```python
from build123d import *

# Parameters (mm, degrees)
SKETCH1_R           = 11
SKETCH1_R_2         = 1.6
BOSS_EXTRUDE1_DEPTH = 5.5
SKETCH2_R           = 3.25
BOSS_EXTRUDE3_DEPTH = 9
CUT_EXTRUDE2_START  = -8
CUT_EXTRUDE2_DEPTH  = 8
SKETCH5_R           = 1.5
CUT_EXTRUDE3_DEPTH  = 22.266170318
CHAMFER1_SIZE       = 1.25
CHAMFER1_SIZE2      = 0.721687836


with BuildPart() as part:
    # Sketch1 → Boss-Extrude1 (new body)
    with BuildSketch(Plane(origin=(0, 0, 0), x_dir=(1, 0, 0), z_dir=(0, 1, 0))):
        with Locations(Location((0, 0, 0), (0, 0, 270))):
            Circle(SKETCH1_R)
        with Locations(Location((0, 7.9, 0), (0, 0, 270))):
            Circle(SKETCH1_R_2, mode=Mode.SUBTRACT)
        with Locations(Location((7.9, 0, 0), (0, 0, 270))):
            Circle(SKETCH1_R_2, mode=Mode.SUBTRACT)
        with Locations(Location((0, -7.9, 0), (0, 0, 270))):
            Circle(SKETCH1_R_2, mode=Mode.SUBTRACT)
        with Locations(Location((-7.9, 0, 0), (0, 0, 270))):
            Circle(SKETCH1_R_2, mode=Mode.SUBTRACT)
    extrude(amount=BOSS_EXTRUDE1_DEPTH)

    # Sketch2 → Boss-Extrude3 (add)
    with BuildSketch(Plane(origin=(0, 5.5, 0), x_dir=(1, 0, 0), z_dir=(0, 1, 0))):
        with Locations(Location((0, 0, 0), (0, 0, 270))):
            Circle(SKETCH2_R)
    extrude(amount=BOSS_EXTRUDE3_DEPTH)

    # Sketch4 → Cut-Extrude2 (cut)
    with BuildSketch(Plane(origin=(0, 14.5, 0), x_dir=(1, 0, 0), z_dir=(0, 1, 0)).offset(CUT_EXTRUDE2_START)):
        with BuildLine():
            Line((2.5, -2.076655966), (-2.5, -2.076655966))
            ThreePointArc((-2.5, -2.076655966), (0, -3.25), (2.5, -2.076655966))
        make_face()
    extrude(amount=CUT_EXTRUDE2_DEPTH, mode=Mode.SUBTRACT)

    # Sketch5 → Cut-Extrude3 (cut, through all)
    with BuildSketch(Plane(origin=(0, 14.5, 0), x_dir=(1, 0, 0), z_dir=(0, 1, 0))):
        with Locations(Location((0, 0, 0), (0, 0, 270))):
            Circle(SKETCH5_R)
    extrude(amount=-CUT_EXTRUDE3_DEPTH, mode=Mode.SUBTRACT)

    # Chamfer1
    chamfer1_edges = [part.edges().sort_by_distance(p)[0] for p in [
        (0, 0, -1.5),
    ]]
    chamfer1_side = [part.faces().sort_by_distance(p)[0] for p in [
        (0, 0, -10.688873016),
    ]]
    chamfer(chamfer1_edges, length=CHAMFER1_SIZE, length2=CHAMFER1_SIZE2, reference=chamfer1_side[0])


solid = part.part
```
Geometry check sheet. Reference: the model listing, model coordinates, mm. A direction names the side the tool comes from. Give positions to 0.01 mm unless a question says otherwise; leave off trailing zeros. Loops run counter-clockwise (first coordinate to the right, second up) from the corner with the lowest first, then second, coordinate; pieces in that order, holes last. Notation, with made-up numbers: M 14.5,66.5 L 55.5,66.5 A11 cw 55.5,86.5 Z; hole C 61.5,6 d5. An arc over 180 degrees is marked long. Write item = value, one per line.
(1) Sectioned sample at A-A, the plane x = 0. Record the cut outline in (y, z).
Answer below:
outline = M 0,-11 L 5.5,-11 L 5.5,-9.5 L 0,-9.5 Z; M 0,-6.3 L 5.5,-6.3 L 5.5,-3.25 L 14.5,-3.25 L 14.5,-1.5 L 0.72,-1.5 L 0,-2.75 Z; M 0,2.75 L 0.72,1.5 L 14.5,1.5 L 14.5,2.08 L 6.5,2.08 L 6.5,3.25 L 5.5,3.25 L 5.5,6.3 L 0,6.3 Z; M 0,9.5 L 5.5,9.5 L 5.5,11 L 0,11 Z
(2) Tool access check on faces 1 (the face through (0, 10, 2.077)), 2 (the face through (9.25, 2.71, 0.86)), 3 (the face through (-2, 5.5, -3)). Record the directions out of +Z, -Z, +X, -X, +Y, -Y that give a thin tool (end or side, any length) a straight path to the whole face; none if there is none.
Answer below:
face_1 = +Z, +X, -X, +Y
face_2 = +Y, -Y
face_3 = +Y
(3) Sectioned sample at D-D, the plane x = -7.9. Record the cut outline in (y, z).
Answer below:
outline = M 0,-7.65 L 5.5,-7.65 L 5.5,-1.6 L 0,-1.6 Z; M 0,1.6 L 5.5,1.6 L 5.5,7.65 L 0,7.65 Z
(4) Release check for a two-part mould opening along Z. For faces 4 (the face through (-0.61, 2.71, 9.38)), 5 (the face through (0, 6.5, 3)), 6 (the face through (0.143, 9.937, -3.247)) record: released by +Z, released by -Z, zero draft, split by the parting line, or undercut.
Answer below:
face_4 = undercut
face_5 = zero draft
face_6 = split by the parting line
(5) Gauge pin test, flat ends, axial feed: pin 1 Ø6 at (x, y) = (3, 11.5) entering from +Z; pin 2 Ø1 at (x, z) = (-5, -0.5) entering from -Y; pin 3 Ø3 at (x, y) = (-0.5, 7.5) entering from +Z; pin 4 Ø5 at (x, y) = (-3.5, 3) entering from -Z. Record the tip position at first contact, or that the pin passes through.
Answer below:
pin_1 = 2.08
pin_2 = 0
pin_3 = 3.25
pin_4 = -10.95
(6) Sectioned sample at B-B, the plane z = 0. Record the cut outline in (x, y), plus the area to 3 significant figures.
Answer below:
outline = M -11,0 L -9.5,0 L -9.5,5.5 L -11,5.5 Z; M -6.3,0 L -2.75,0 L -1.5,0.72 L -1.5,14.5 L -3.25,14.5 L -3.25,5.5 L -6.3,5.5 Z; M 1.5,0.72 L 2.75,0 L 6.3,0 L 6.3,5.5 L 3.25,5.5 L 3.25,14.5 L 1.5,14.5 Z; M 9.5,0 L 11,0 L 11,5.5 L 9.5,5.5 Z
area = 99.9 mm2
(7) Sectioned sample at C-C, the plane z = -7.9. Record the cut outline in (x, y).
Answer below:
outline = M -7.65,0 L -1.6,0 L -1.6,5.5 L -7.65,5.5 Z; M 1.6,0 L 7.65,0 L 7.65,5.5 L 1.6,5.5 Z
(8) Material ranges on line 1 (X direction, y = 3.45, z = 0); line 2 (Y direction, x = 3.5, z = -6); line 3 (Z direction, x = 0.75, y = 1.5), recorded low to high. Write a range as [from, to].
Answer below:
line_1 = [-11, -9.5], [-6.3, -1.5], [1.5, 6.3], [9.5, 11]
line_2 = [0, 5.5]
line_3 = [-10.97, -9.31], [-6.49, -1.3], [1.3, 6.49], [9.31, 10.97]
